Input: part model. Units: mm. Frame: model coordinates. Face numbers are marked on the shaded views. A direction names the side the tool comes from. Coordinates: 2 decimals unless noted, no trailing zeros. Order: outer loops, then holes, each group sorted by start corner. A loop starts at its lowest first (then second) coordinate and runs counter-clockwise, first axis right, second up. Notation, with made-up numbers: (28, 20.25) -> (39, 20.25) arc R19 ccw to (39, 47.25) -> close; hole circle Ø8 at (61, 29). An arc over 180 degrees is marked (long way). Write each question's results on one line, items separated by ' | '.
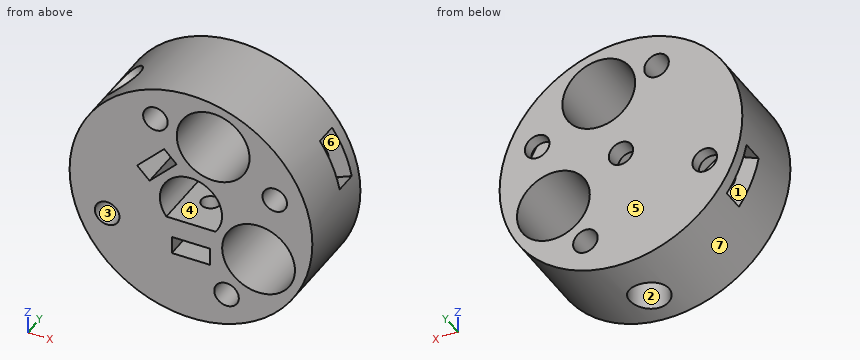
```python
from build123d import *

# Parameters (mm, degrees)
SKETCH1_R               = 20
BOSS_EXTRUDE1_DEPTH     = 7.5
SKETCH4_R               = 5.125
CUT_EXTRUDE2_DEPTH      = 12.15
SKETCH5_R               = 2
CUT_EXTRUDE3_DEPTH      = 1
CUT_EXTRUDE3_DEPTH_BACK = 16
SKETCH15_W              = 8.1
SKETCH15_H              = 1.984438744
BOSS_EXTRUDE3_DEPTH     = 12.15
SKETCH2_R               = 2.025
CUT_EXTRUDE1_DEPTH      = 16
CIRPATTERN1_COUNT       = 4
SKETCH6_R               = 1.525
CUT_EXTRUDE4_DEPTH      = 21
CUT_EXTRUDE5_START      = -20
SKETCH7_R               = 3.25
CUT_EXTRUDE5_DEPTH      = 8
CUT_EXTRUDE11_START     = -6.5
CUT_EXTRUDE11_DEPTH     = 2.9
CIRPATTERN2_COUNT       = 2
CIRPATTERN2_ANGLE       = 135
CUT_EXTRUDE7_START      = 5.5
CUT_EXTRUDE7_DEPTH      = 3.8
CIRPATTERN3_COUNT       = 2
CUT_EXTRUDE12_START     = -16.0000001
SKETCH10_R              = 6
CUT_EXTRUDE12_DEPTH     = 17.0000002
CIRPATTERN4_COUNT       = 2
CIRPATTERN4_ANGLE       = 100


with BuildPart() as part:
    # Sketch1 → Boss-Extrude1 (new body, symmetric)
    with BuildSketch(Plane(origin=(0, 0, 0), x_dir=(1, 0, 0), z_dir=(0, 1, 0))):
        Circle(SKETCH1_R)
    extrude(amount=BOSS_EXTRUDE1_DEPTH, both=True)

    # Sketch4 → Cut-Extrude2 (cut)
    with BuildSketch(Plane.XZ.offset(7.5)):
        Circle(SKETCH4_R)
    extrude(amount=-CUT_EXTRUDE2_DEPTH, mode=Mode.SUBTRACT)

    # Sketch5 → Cut-Extrude3 (cut, two sides)
    with BuildSketch(Plane(origin=(0, 7.5, 0), x_dir=(1, 0, 0), z_dir=(0, 1, 0))) as cut_extrude3_sk:
        Circle(SKETCH5_R)
    extrude(amount=CUT_EXTRUDE3_DEPTH, mode=Mode.SUBTRACT)
    extrude(cut_extrude3_sk.sketch, amount=-CUT_EXTRUDE3_DEPTH_BACK, mode=Mode.SUBTRACT)

    # Sketch15 → Boss-Extrude3 (add)
    with BuildSketch(Plane.XZ.offset(7.5)):
        with Locations((0, -4.132780628)):
            Rectangle(SKETCH15_W, SKETCH15_H)
    extrude(amount=-BOSS_EXTRUDE3_DEPTH)

    # Sketch2 → Cut-Extrude1 (cut, through all)
    with BuildSketch(Plane(origin=(0, 7.5, 0), x_dir=(1, 0, 0), z_dir=(0, 1, 0))):
        with Locations((-13.807572802, 5.860966927)):
            Circle(SKETCH2_R)
    cut_extrude1 = extrude(amount=-CUT_EXTRUDE1_DEPTH, mode=Mode.SUBTRACT)

    # CirPattern1: Cut-Extrude1 ×4 about axis
    cirpattern1_axis = Axis((0, 0, 0), (0, 1, 0))
    for i in range(1, CIRPATTERN1_COUNT):
        add(cut_extrude1.rotate(cirpattern1_axis, i * 360 / CIRPATTERN1_COUNT), mode=Mode.SUBTRACT)

    # Sketch6 → Cut-Extrude4 (cut, through all)
    with BuildSketch(Plane.XY):
        with Locations((0, -1.35)):
            Circle(SKETCH6_R)
    cut_extrude4 = extrude(amount=-CUT_EXTRUDE4_DEPTH, mode=Mode.SUBTRACT)

    # Sketch7 → Cut-Extrude5 (cut)
    with BuildSketch(Plane.XY.offset(CUT_EXTRUDE5_START)):
        with Locations((0, -1.35)):
            Circle(SKETCH7_R)
    cut_extrude5 = extrude(amount=CUT_EXTRUDE5_DEPTH, mode=Mode.SUBTRACT)

    # Sketch9 → Cut-Extrude11 (cut)
    with BuildSketch(Plane.XY.offset(CUT_EXTRUDE11_START)):
        Polygon((3.15, -3.168653348), (3.15, 0.468653348), (0, 2.287306696), (-3.15, 0.468653348), (-3.15, -3.168653348), (-3.15, -7.685074736), (3.15, -7.685074736), align=None)
    cut_extrude11 = extrude(amount=-CUT_EXTRUDE11_DEPTH, mode=Mode.SUBTRACT)

    # CirPattern2: Cut-Extrude4, Cut-Extrude5, Cut-Extrude11 ×2 about axis
    cirpattern2_axis = Axis((0, 0, 0), (0, 1, 0))
    for i in range(1, CIRPATTERN2_COUNT):
        add(cut_extrude4.rotate(cirpattern2_axis, i * CIRPATTERN2_ANGLE / (CIRPATTERN2_COUNT - 1)), mode=Mode.SUBTRACT)
        add(cut_extrude5.rotate(cirpattern2_axis, i * CIRPATTERN2_ANGLE / (CIRPATTERN2_COUNT - 1)), mode=Mode.SUBTRACT)
        add(cut_extrude11.rotate(cirpattern2_axis, i * CIRPATTERN2_ANGLE / (CIRPATTERN2_COUNT - 1)), mode=Mode.SUBTRACT)

    # Sketch8 → Cut-Extrude7 (cut)
    with BuildSketch(Plane(origin=(0, 0, 0), x_dir=(1, 0, 0), z_dir=(0, 1, 0)).offset(CUT_EXTRUDE7_START)):
        Polygon((-9.396506885, 3.988580533), (-9.98050566, 8.744868872), (-14.391571577, 10.617255266), (-19.569899143, 12.815324908), (-22.81296751, 5.175134625), (-17.634639943, 2.977064983), (-13.223574027, 1.104678588), align=None)
    cut_extrude7 = extrude(amount=-CUT_EXTRUDE7_DEPTH, mode=Mode.SUBTRACT)

    # CirPattern3: Cut-Extrude7 ×2 about axis
    cirpattern3_axis = Axis((0, 0, 0), (0, 1, 0))
    for i in range(1, CIRPATTERN3_COUNT):
        add(cut_extrude7.rotate(cirpattern3_axis, i * 360 / CIRPATTERN3_COUNT), mode=Mode.SUBTRACT)

    # Sketch10 → Cut-Extrude12 (cut)
    with BuildSketch(Plane(origin=(0, 7.5, 0), x_dir=(1, 0, 0), z_dir=(0, 1, 0)).offset(CUT_EXTRUDE12_START)):
        with Locations((3.654646309, -11.95380945)):
            Circle(SKETCH10_R)
    cut_extrude12 = extrude(amount=CUT_EXTRUDE12_DEPTH, mode=Mode.SUBTRACT)

    # CirPattern4: Cut-Extrude12 ×2 about axis
    cirpattern4_axis = Axis((0, 7.5, 0), (0, 1, 0))
    for i in range(1, CIRPATTERN4_COUNT):
        add(cut_extrude12.rotate(cirpattern4_axis, i * CIRPATTERN4_ANGLE / (CIRPATTERN4_COUNT - 1)), mode=Mode.SUBTRACT)


solid = part.part
```
(1) Line query: line 1 along X through (y, z) = (6.75, -1); line 2 along X through (y, z) = (-0.5, 2.5); line 3 along Z through (x, y) = (14, 6). Output: solid intervals per line, ascending. Write a range as from..to.
Return value:
line 1: -19.97..-1.73, 1.73..7.38, 14.9..19.97 | line 2: -19.84..-6.95, -6.69..-4.47, 4.47..19.84 | line 3: -14.28..-10.95, -0.4..3.85, 7.88..14.28
(2) Cut plane C-C, the plane z = -2.5. Return loops of the section in (x, y).
Return value:
outline: (-19.84, -7.5) -> (-4.47, -7.5) -> (-4.47, 4.65) -> (4.47, 4.65) -> (4.47, -7.5) -> (6.05, -7.5) -> (6.05, 7.5) -> (-19.84, 7.5) -> close; (16.23, -7.5) -> (19.84, -7.5) -> (19.84, 7.5) -> (16.23, 7.5) -> close; hole (-16.51, 1.7) -> (-11.37, 1.7) -> (-11.37, 5.5) -> (-16.51, 5.5) -> close
(3) Pin query (flat end, axial travel): P1, Ø6.5, axis at x = 0.5, y = -0.5, coming from the +Z side; P2, Ø4, axis at x = 10, y = -0.5, coming from the +Z side; P3, Ø1, axis at x = 8, y = 2.5, coming from the -Z side. Return the tip coordinate at first contact, or that it passes through.
Return value:
P1: z = 20 | P2: z = 18.33 | P3: z = -18.54
(4) Mould query, pull axis Z, two halves, no side actions, for the marked faces 5, 6 and 7. Classes: +Z half, -Z half, draft (parallel to the pull), parting line (faces both ways), or undercut.
Return value:
face 5: draft | face 6: undercut | face 7: parting line
(5) Reachability of the marked faces 1, 2, 3 and 4 from +Z, -Z, +X, -X, +Y, -Y: full face, straight path, thin tool, end or side. Return the list, or none.
Return value:
face 1: none | face 2: -Z | face 3: +Y, -Y | face 4: -Y
(6) Cut plane B-B, the plane y = 1. Count the separate pieces of the cut face and the enclosed holes in it, plus the area to 3 significant figures.
Return value:
separate pieces: 1 | enclosed holes: 9 | area: 810 mm2
(7) Cut plane A-A, the plane z = -15. Return loops of the section in (x, y).
Return value:
outline: (-13.23, -7.5) -> (4.22, -7.5) -> (4.22, 7.5) -> (-13.23, 7.5) -> close; (7.5, -7.5) -> (13.23, -7.5) -> (13.23, 7.5) -> (7.5, 7.5) -> close; hole circle Ø6.5 at (0, -1.35)
